```python
from build123d import *

# Parameters (mm, degrees)
BOSS_EXTRUDE1_DEPTH = 11
SKETCH3_W           = 22
SKETCH3_H           = 3
BOSS_EXTRUDE2_DEPTH = 15.7
BOSS_EXTRUDE3_DEPTH = 5
SKETCH5_R           = 1.75
CUT_EXTRUDE1_DEPTH  = 36.096650541
SKETCH6_W           = 9
SKETCH6_H           = 9
BOSS_EXTRUDE4_DEPTH = 5
SKETCH7_R           = 2.25
CUT_EXTRUDE2_DEPTH  = 37.945027801
FILLET1_R           = 1


with BuildPart() as part:
    # Sketch1 → Boss-Extrude1 (new, symmetric)
    with BuildSketch(Plane(origin=(0, 0, 0), x_dir=(0, 0, -1), z_dir=(1, 0, 0))):
        Polygon((-13.0089, 0), (13.0089, 0), (13.0089, 8.5), (5.7589, 8.5), (5.7589, 7), (-5.7589, 7), (-5.7589, 8.5), (-13.0089, 8.5), align=None)
    extrude(amount=BOSS_EXTRUDE1_DEPTH, both=True)

    # Sketch3 → Boss-Extrude2 (add)
    with BuildSketch(Plane.XZ):
        with Locations((0, -14.5089)):
            Rectangle(SKETCH3_W, SKETCH3_H)
        with Locations((0, 14.5089)):
            Rectangle(SKETCH3_W, SKETCH3_H)
    extrude(amount=-BOSS_EXTRUDE2_DEPTH)

    # Sketch4 → Boss-Extrude3 (add)
    with BuildSketch(Plane(origin=(11, 0, 0), x_dir=(0, 0, -1), z_dir=(1, 0, 0))):
        Polygon((-8.8, 15.7), (-16.0089, 15.7), (-16.0089, 0), (16.0089, 0), (16.0089, 15.7), align=None)
    extrude(amount=BOSS_EXTRUDE3_DEPTH)

    # Sketch5 → Cut-Extrude1 (cut, through all)
    with BuildSketch(Plane(origin=(16, 0, 0), x_dir=(0, 0, -1), z_dir=(1, 0, 0))):
        with Locations((-10.5, 11)):
            Circle(SKETCH5_R)
        with Locations((10.5, 11)):
            Circle(SKETCH5_R)
    extrude(amount=-CUT_EXTRUDE1_DEPTH, mode=Mode.SUBTRACT)

    # Sketch6 → Boss-Extrude4 (add)
    with BuildSketch(Plane.XZ):
        with Locations((20.5, 0)):
            Rectangle(SKETCH6_W, SKETCH6_H)
        with Locations((11.5, -20.5089)):
            Rectangle(SKETCH6_W, SKETCH6_H)
    extrude(amount=-BOSS_EXTRUDE4_DEPTH)

    # Sketch7 → Cut-Extrude2 (cut, through all)
    with BuildSketch(Plane(origin=(0, 5, 0), x_dir=(1, 0, 0), z_dir=(0, 1, 0))):
        with Locations(Location((20.5, 0, 0), (0, 0, 270))):
            Circle(SKETCH7_R)
        with Locations(Location((11.5, 20.5089, 0), (0, 0, 270))):
            Circle(SKETCH7_R)
    extrude(amount=-CUT_EXTRUDE2_DEPTH, mode=Mode.SUBTRACT)

    # Fillet1
    fillet1_edges = [part.edges().sort_by_distance(p)[0] for p in [
        (0, 8.5, 5.7589),
        (0, 8.5, -5.7589),
        (0, 15.7, -13.0089),
        (11, 12.1, -13.0089),
        (11, 12.1, 13.0089),
        (0, 15.7, 13.0089),
        (11, 15.7, 0),
        (25, 5, 0),
        (11.5, 5, -25.0089),
    ]]
    fillet(fillet1_edges, radius=FILLET1_R)


solid = part.part
```
Work out the finished part from the listing and answer in its coordinate system (mm). A direction names the side the tool comes from. Coordinates: 2 decimals unless noted, no trailing zeros. Write each loop counter-clockwise with the first axis right and the second up, starting at its lowest first coordinate (ties: lowest second). Pieces come first, ordered by that corner, then holes. Notation, with made-up numbers: (-16.5, 87) - (13.5, 87) arc R18 ccw to (13.5, 121) - close; hole circle Ø8 at (29, -9.75). An arc over 180 degrees is marked (long way). Answer as a JSON object with one key per item and string values.
Q1. Find section C-C (x = 4.5). Write down the section's boundary in (y, z).
Results list:
{"outline": "(0, -16.01) - (15.7, -16.01) - (15.7, -14.01) arc R1 ccw to (14.7, -13.01) - (8.5, -13.01) - (8.5, -6.76) arc R1 ccw to (7.5, -5.76) - (7, -5.76) - (7, 5.76) - (7.5, 5.76) arc R1 ccw to (8.5, 6.76) - (8.5, 13.01) - (14.7, 13.01) arc R1 ccw to (15.7, 14.01) - (15.7, 16.01) - (0, 16.01) - close"}
Q2. Find section A-A (x = 20.5). Write down the section's boundary in (y, z), plus the area to 3 significant figures.
Results list:
{"outline": "(0, -4.5) - (5, -4.5) - (5, -2.25) - (0, -2.25) - close; (0, 2.25) - (5, 2.25) - (5, 4.5) - (0, 4.5) - close", "area": "22.5 mm^2"}
Q3. Consider L1, parallel to Z at x = 14.7, y = 11; L2, parallel to Z at x = -3, y = 7.5; L3, parallel to Y at x = 13.25, z = 10.5. Determine where each line is inside the solid, lowest interval first. Write a range as from..to.
Results list:
{"L1": "z = -16.01..-12.25, -8.75..8.75, 12.25..16.01", "L2": "z = -16.01..-5.76, 5.76..16.01", "L3": "y = 0..9.25, 12.75..15.7"}
Q4. Find section D-D (z = -22). Write down the section's boundary in (x, y), plus the area to 3 significant figures.
Results list:
{"outline": "(7, 0) - (9.82, 0) - (9.82, 5) - (7, 5) - close; (13.18, 0) - (16, 0) - (16, 5) - (13.18, 5) - close", "area": "28.2 mm^2"}
Q5. Find section B-B (z = -10.5). Write down the section's boundary in (x, y), plus the area to 3 significant figures.
Results list:
{"outline": "(-11, 0) - (16, 0) - (16, 9.25) - (11, 9.25) - (11, 8.5) - (-11, 8.5) - close; (11, 12.75) - (16, 12.75) - (16, 15.7) - (12, 15.7) arc R1 ccw to (11, 14.7) - close", "area": "248 mm^2"}
Q6. Given pin 1 Ø1.5 at (x, y) = (7.5, 8) entering from -Z; pin 2 Ø3 at (x, z) = (-5, 10) entering from +Y; pin 3 Ø4.5 at (y, z) = (11, -10.5) entering from +X, each flat-ended and moving along its own axis, determine where each tip first touches the part or whether it passes through.
Results list:
{"pin 1": "stops at z = -16.01", "pin 2": "stops at y = 8.5", "pin 3": "stops at x = 16"}
Q7. Which of the six approach directions +Z, -Z, +X, -X, +Y, -Y give full straight-line access (tool end or side, diameter ignored) to faces 4 (the flat face through (0, 8.5, -10)), 5 (the flat face through (18, 5, 0)), 6 (the flat face through (20, 2, -4.5)), 7 (the cylindrical face through (18.304, 2.535, -0.488)), 8 (the flat face through (7, 2, -21))?
Results list:
{"face 4": "-X, +Y", "face 5": "+Z, -Z, +X, +Y", "face 6": "-Z, +X, +Y, -Y", "face 7": "+Y, -Y", "face 8": "-Z, -X, +Y, -Y"}
Q8. For a pull along X with two mould halves and no side action, classify faces 1 (the flat face through (20, 2, 4.5)), 2 (the cylindrical face through (10.699, 13.313, 12.724)), 3 (the cylindrical face through (13.02, 2.54, -22.17)) as pulls with the +X half, pulls with the -X half, needs draft (parallel to the pull), parting line crosses it, or undercut.
Results list:
{"face 1": "needs draft", "face 2": "pulls with the -X half", "face 3": "undercut"}
